Read the model definition and answer for the solid it produces. Units are mm, in the model's axes. A direction names the side the tool comes from. Give positions to 0.01 mm unless a question says otherwise; leave off trailing zeros. Loops run counter-clockwise (first coordinate to the right, second up) from the corner with the lowest first, then second, coordinate; pieces in that order, holes last. Notation, with made-up numbers: (86, -32) - (128, -32) arc R20 cw to (128, -17) - close; hole circle Ø8 at (14, -33). An arc over 180 degrees is marked (long way). Write each question's results on one line, items separated by ' | '. Start each with the question number.
Q1. Given pin 1 (12 mm diameter, centred on x = 22, y = -157, fed in from +Z); pin 2 (1.5 mm diameter, centred on x = 35.5, y = -22, fed in from -Z); pin 3 (10 mm diameter, centred on x = 34.5, z = -73, fed in from -Y), each flat-ended and moving along its own axis, determine where each tip first touches the part or whether it passes through.
Q2. Determine the mould class of faces 5 (the flat face through (74, -187, -63)), 6 (the cylindrical face through (48.025, -3.517, -79.923)), 7 (the cylindrical face through (57.07, 122.914, -160.3)) for opening direction Z: +Z half, -Z half, draft (parallel to the pull), parting line (faces both ways), or undercut.
Q3. For faces 1 (the flat face through (40, 24, 1)), 2 (the flat face through (170, 36, -42)), 3 (the flat face through (85, 71, 0)), 4 (the flat face through (52, -171, -109)), determine the directions among +Z, -Z, +X, -X, +Y, -Y from which every point of the face is accessible in a straight line to the end or side of a thin tool.
Q4. The part is cut by section A-A, the plane x = 113. Write down the section's boundary in (y, z).
Q5. Find the intervals of material crossed by line 1 (Y direction, x = 55, z = 0); line 2 (Z direction, x = 22.5, y = -71); line 3 (X direction, y = -2, z = -37), in increasing order. Write a range as from..to.
Q6. The part is cut by section B-B, the plane x = 17.5. Write down the section's boundary in (y, z).
```python
from build123d import *

# Parameters (mm, degrees)
FILLET1_R = 10


with BuildPart() as part:
    # Sketch1 → Revolve1 (revolve)
    with BuildSketch(Plane.XY, mode=Mode.PRIVATE) as revolve1_sk:
        with BuildLine():
            Line((170, 55), (130, 55))
            Line((130, 55), (130, 21.009993912))
            Line((130, 21.009993912), (40, 21.009993912))
            Line((40, 21.009993912), (40, 55))
            Line((40, 55), (0, 55))
            Line((0, 55), (0, 180))
            ThreePointArc((0, 180), (23.569740978, 192.840057103), (45, 209))
            Line((45, 209), (52, 209))
            Line((52, 209), (52, 202))
            Line((52, 202), (62, 202))
            Line((62, 202), (62, 209))
            Line((62, 209), (74, 209))
            Line((74, 209), (74, 197))
            Line((74, 197), (44, 197))
            Line((44, 197), (10, 170))
            Line((10, 170), (10, 80))
            Line((10, 80), (85, 80))
            Line((85, 80), (85, 70))
            Line((85, 70), (170, 70))
            Line((170, 70), (170, 55))
        make_face()
    revolve(revolve1_sk.sketch.rotate(Axis((0, 0, 0), (1, 0, 0)), 90), axis=Axis((0, 0, 0), (1, 0, 0)))

    # Fillet1
    fillet1_edges = [part.edges().sort_by_distance(p)[0] for p in [
        (0, 0, -180),
        (45, 0, -209),
    ]]
    fillet(fillet1_edges, radius=FILLET1_R)


solid = part.part
```
Check sheet entries:
1) pin 1: stops at z = 120.58 | pin 2: stops at z = -200.6 | pin 3: stops at y = -191.28
2) face 5: draft | face 6: undercut | face 7: parting line
3) face 1: -X | face 2: +Z, -Z, +X, +Y, -Y | face 3: +X | face 4: none
4) outline: circle Ø140 at (0, 0); hole circle Ø42.02 at (0, 0)
5) line 1: y = -202..-197, -80..-21.01, 21.01..80, 197..202 | line 2: z = -178.56..-165.33, -36.86..36.86, 165.33..178.56 | line 3: x = 40..130
6) outline: circle Ø378.19 at (0, 0); circle Ø160 at (0, 0); hole circle Ø351.91 at (0, 0); hole circle Ø110 at (0, 0)
